from build123d import *

# Parameters (mm, degrees)
BOSS_EXTRUDE1_DEPTH = 2.5
SKETCH5_W           = 3
SKETCH5_H           = 2.5
CUT_EXTRUDE2_DEPTH  = 10
SKETCH6_W           = 3
SKETCH6_H           = 2.5
CUT_EXTRUDE3_DEPTH  = 10
SKETCH7_W           = 3
SKETCH7_H           = 2.5
CUT_EXTRUDE4_DEPTH  = 10


with BuildPart() as part:
    # Sketch1 → Boss-Extrude1 (new body)
    with BuildSketch(Plane(origin=(0, 0, 0), x_dir=(1, 0, 0), z_dir=(0, 1, 0))):
        Polygon((8.581310361, -0.009375041), (4.251183342, 7.490624959), (-8.409070695, 7.490624959), (-12.739197714, -0.009375041), (-8.409070695, -7.509375041), (4.251183342, -7.509375041), align=None)
    extrude(amount=BOSS_EXTRUDE1_DEPTH)

    # Sketch5 → Cut-Extrude2 (cut)
    with BuildSketch(Plane.XY.offset(7.509375041)):
        with Locations((-6.909070695, 1.25)):
            Rectangle(SKETCH5_W, SKETCH5_H)
    extrude(amount=-CUT_EXTRUDE2_DEPTH, mode=Mode.SUBTRACT)

    # Sketch6 → Cut-Extrude3 (cut)
    with BuildSketch(Plane.XY.offset(7.509375041)):
        with Locations((2.751183342, 1.25)):
            Rectangle(SKETCH6_W, SKETCH6_H)
    extrude(amount=-CUT_EXTRUDE3_DEPTH, mode=Mode.SUBTRACT)

    # Sketch7 → Cut-Extrude4 (cut)
    with BuildSketch(Plane(origin=(0, 0, -7.490624959), x_dir=(-1, 0, 0), z_dir=(0, 0, -1))):
        with Locations((2.078816658, 1.25)):
            Rectangle(SKETCH7_W, SKETCH7_H)
    extrude(amount=-CUT_EXTRUDE4_DEPTH, mode=Mode.SUBTRACT)


solid = part.part
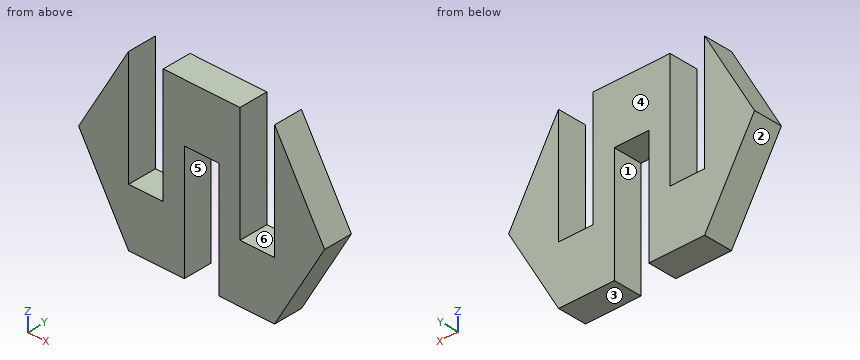
Geometry: final body of the model. Coordinates: model frame, mm. Face numbers are marked on the shaded views. A direction names the side the tool comes from. Coordinates: 2 decimals unless noted, no trailing zeros. Order: outer loops, then holes, each group sorted by start corner. A loop starts at its lowest first (then second) coordinate and runs counter-clockwise, first axis right, second up.
1) Ray query, probe 1 along X at (y, z) = (0.7, 3.75); probe 2 along X at (y, z) = (1.4, -1.5); probe 3 along X at (y, z) = (1.3, 7). Return the intervals inside material, ascending.
Result sheet:
probe 1: x = -10.58 to -8.41, -5.41 to 1.25, 4.25 to 6.42
probe 2: x = -11.87 to -8.41, -5.41 to -3.58, -0.58 to 1.25, 4.25 to 7.71
probe 3: x = -8.7 to -8.41, -5.41 to 1.25, 4.25 to 4.55
2) Section B-B (y = 1.2). Return loops of the section in (x, z).
Result sheet:
outline: (-12.74, 0.01) - (-8.41, -7.49) - (-3.58, -7.49) - (-3.58, 2.51) - (-0.58, 2.51) - (-0.58, -7.49) - (4.25, -7.49) - (8.58, 0.01) - (4.25, 7.51) - (4.25, -2.49) - (1.25, -2.49) - (1.25, 7.51) - (-5.41, 7.51) - (-5.41, -2.49) - (-8.41, -2.49) - (-8.41, 7.51) - close
3) Draft query along X for the marked faces 1, 2 and 3. Return one class per face: released by +X, released by -X, zero draft, split by the parting line, or undercut.
Result sheet:
face 1: undercut
face 2: released by -X
face 3: zero draft
4) First-contact query: P1, Ø1.2, axis at x = -2.5, y = 1, coming from the -Z side; P2, Ø1.5, axis at y = 2, z = -2.5, coming from the -X side; P3, Ø0.8, axis at y = 1.5, z = 3, coming from the -X side. Flat tips, straight axial feed; report the tip coordinate or a pass-through.
Result sheet:
P1: stops at z = 2.51
P2: stops at x = -11.72
P3: stops at x = -11.24
5) Section A-A (z = -2). Return loops of the section in (x, y), then the cut area to 3 significant figures.
Result sheet:
outline: (-11.58, 0) - (-8.41, 0) - (-8.41, 2.5) - (-11.58, 2.5) - close; (-5.41, 0) - (-3.58, 0) - (-3.58, 2.5) - (-5.41, 2.5) - close; (-0.58, 0) - (1.25, 0) - (1.25, 2.5) - (-0.58, 2.5) - close; (4.25, 0) - (7.42, 0) - (7.42, 2.5) - (4.25, 2.5) - close
area: 25.0 mm2
6) Set-up query: the marked faces 4, 5 and 6. Return all of +Z, -Z, +X, -X, +Y, -Y with unobstructed straight access to the full face (end or side cutting, diameter ignored); none if empty.
Result sheet:
face 4: +Z, -Z, +X, -X, +Y
face 5: -Z, +Y, -Y
face 6: +Z, +Y, -Y
7) Section C-C (z = -4). Return loops of the section in (x, y), then the cut area to 3 significant figures.
Result sheet:
outline: (-10.42, 0) - (-3.58, 0) - (-3.58, 2.5) - (-10.42, 2.5) - close; (-0.58, 0) - (6.27, 0) - (6.27, 2.5) - (-0.58, 2.5) - close
area: 34.2 mm2
8) Section D-D (z = 5.75). Return loops of the section in (x, y), then the cut area to 3 significant figures.
Result sheet:
outline: (-9.42, 0) - (-8.41, 0) - (-8.41, 2.5) - (-9.42, 2.5) - close; (-5.41, 0) - (1.25, 0) - (1.25, 2.5) - (-5.41, 2.5) - close; (4.25, 0) - (5.27, 0) - (5.27, 2.5) - (4.25, 2.5) - close
area: 21.7 mm2
